Autodesk Fusion 360 part; units mm, degrees
sketch "スケッチ1" plane through (0, 0, 0) normal (0, 1, 0) x (1, 0, 0)
  line L0 (-48, 0) -> (48, 0)
  line L1 (-50.0166, 2) -> (-50.0166, 30)
  line L2 (-48, 32) -> (-40, 32)
  line L3 (-40, 32) -> (-40, 35)
  line L4 (-38, 37) -> (-9.5, 37)
  line L5 (50, 2) -> (50, 30)
  line L6 (48, 32) -> (40, 32)
  line L7 (40, 32) -> (40, 35)
  line L8 (38, 37) -> (9.5, 37)
  line L9 (-7.5, 32) -> (7.5, 32)
  arc A0 (-38, 37) -> (-40, 35) centre (-38, 35) ccw
  line L10 (-7.5, 35.0262) -> (-7.5, 32)
  line L11 (7.4996, 35.0262) -> (7.5, 32)
  arc A1 (-48, 32) -> (-50.0166, 30) centre (-48, 29.9833) ccw
  arc A2 (-7.5, 35.0262) -> (-9.5, 37) centre (-9.5, 34.9998) ccw
  arc A3 (9.5, 37) -> (7.4996, 35.0262) centre (9.5, 34.9994) ccw
  arc A4 (40, 35) -> (38, 37) centre (38, 35) ccw
  arc A5 (50, 30) -> (48, 32) centre (48, 30) ccw
  arc A6 (48, 0) -> (50, 2) centre (48, 2) ccw
  arc A7 (-50.0166, 2) -> (-48, 0) centre (-48.0165, 2) ccw
  dimension "d1" = 96
  dimension "d2" = 28
  dimension "d3" = 8
  dimension "d4" = 28.5
  dimension "d5" = 28
  dimension "d6" = 8
  dimension "d7" = 28.5
extrude "押し出し1" add sketch "スケッチ1" along normal blind 2
Verification items for the finished model (mm, model axes). A direction names the side the tool comes from. Coordinates: 2 decimals unless noted, no trailing zeros. Write each loop counter-clockwise with the first axis right and the second up, starting at its lowest first coordinate (ties: lowest second). Pieces come first, ordered by that corner, then holes. Notation, with made-up numbers: (70.25, 30.5) - (85.25, 30.5) arc R12 ccw to (85.25, 53.5) - close; hole circle Ø8 at (-20.5, -14.5). An arc over 180 degrees is marked (long way). Answer as a JSON object with one key per item and string values.
(1) Tool access check on faces 4 (the flat face through (24, 1, -37)), 5 (the flat face through (40, 1, -33)), 6 (the flat face through (-44, 1, -32)), 7 (the flat face through (0, 1, -32)), 8 (the flat face through (50, 1, -16)). Record the directions out of +Z, -Z, +X, -X, +Y, -Y that give a thin tool (end or side, any length) a straight path to the whole face; none if there is none.
Report:
{"face 4": "-Z, +X, -X, +Y, -Y", "face 5": "-Z, +X, +Y, -Y", "face 6": "-Z, -X, +Y, -Y", "face 7": "-Z, +Y, -Y", "face 8": "+Z, -Z, +X, +Y, -Y"}
(2) Cross-section at A-A on y = 0.6. Record the cut outline in (x, z).
Report:
{"outline": "(-50.02, -30) arc R2.02 ccw to (-48, -32) - (-40, -32) - (-40, -35) arc R2 ccw to (-38, -37) - (-9.5, -37) arc R2 ccw to (-7.5, -35.03) - (-7.5, -32) - (7.5, -32) - (7.5, -35.03) arc R2 ccw to (9.5, -37) - (38, -37) arc R2 ccw to (40, -35) - (40, -32) - (48, -32) arc R2 ccw to (50, -30) - (50, -2) arc R2 ccw to (48, 0) - (-48, 0) arc R2 ccw to (-50.02, -2) - close"}
(3) Mould release check, pull along X, two halves, no side actions. Record for faces 1 (the cylindrical face through (49.4, 0.99, -31.43)), 2 (the flat face through (-7.5, 1, -34)), 3 (the flat face through (-1, 1, 0)): pulls with the +X half, pulls with the -X half, needs draft (parallel to the pull), parting line crosses it, or undercut.
Report:
{"face 1": "pulls with the +X half", "face 2": "undercut", "face 3": "needs draft"}
(4) Cross-section at B-B on x = -6.5. Record the cut outline in (y, z).
Report:
{"outline": "(0, -32) - (2, -32) - (2, 0) - (0, 0) - close"}
(5) Gauge pin test, flat ends, axial feed: pin 1 Ø0.6 at (y, z) = (1, -34) entering from +X; pin 2 Ø0.6 at (y, z) = (1.5, -33.5) entering from -X; pin 3 Ø0.6 at (x, y) = (-1.5, 0.5) entering from -Z. Record the tip position at first contact, or that the pin passes through.
Report:
{"pin 1": "x = 40", "pin 2": "x = -40", "pin 3": "z = -32"}
(6) Thickness scan on line 1 along Z through (x, y) = (46.5, 0.75). Record the ranges inside material, lowest first.
Report:
{"line 1": "-32 to 0"}
